from build123d import *

# Parameters (mm, degrees)
SHELL2_T = -1


with BuildPart() as part:
    # Sketch1 → Revolve3 (revolve)
    with BuildSketch(Plane.XY, mode=Mode.PRIVATE) as revolve3_sk:
        with BuildLine():
            Line((0, 0), (70.170274015, 0))
            ThreePointArc((70.170274015, 0), (74.867019818, 0.813696051), (79.016316154, 3.159940352))
            ThreePointArc((79.016316154, 3.159940352), (83.467476244, 7.068955028), (87.638838201, 11.275255219))
            ThreePointArc((87.638838201, 11.275255219), (93.444928024, 16.921383546), (99.811810502, 21.926605983))
            ThreePointArc((99.811810502, 21.926605983), (122.101594507, 34.410654829), (146.474870989, 42.06763466))
            Line((146.474870989, 42.06763466), (146.474870989, 43.043574036))
            Line((146.474870989, 43.043574036), (0, 43.043574036))
            Line((0, 43.043574036), (0, 0))
        make_face()
    revolve(revolve3_sk.sketch.rotate(Axis((0, 43.043574036, 0), (0, -1, 0)), 90), axis=Axis((0, 43.043574036, 0), (0, -1, 0)))

    # Shell2
    shell2_openings = [part.faces().sort_by_distance(p)[0] for p in [
        (0, 43.043574036, 0),
    ]]
    offset(amount=SHELL2_T, openings=shell2_openings, kind=Kind.INTERSECTION)


solid = part.part
Check sheet for the modelled part. Datum: model origin and axes. Units: mm. Give positions to 0.01 mm unless a question says otherwise; leave off trailing zeros. Loops run counter-clockwise (first coordinate to the right, second up) from the corner with the lowest first, then second, coordinate; pieces in that order, holes last. Notation, with made-up numbers: M 60.25,68 L 107.25,68 A30 cw 107.25,105 Z; hole C 38,7 d8. An arc over 180 degrees is marked long. Answer as a JSON object with one key per item and string values. Group by question number.
Q1. Release check for a two-part mould opening along Z. For faces 1 (the flat face through (-1, 0, 1)), 2 (the flat face through (-1, 1, 1)), 3 (the cylindrical face through (-44, 42.56, 139.71)) record: released by +Z, released by -Z, zero draft, split by the parting line, or undercut.
Q2. Cross-section at A-A on y = 32. Record the cut outline in (x, z).
Q3. Material ranges on line 1 along X through (y, z) = (23, 71); line 2 along Y through (x, z) = (27.5, 20.5); line 3 along X through (y, z) = (28, -30.5), recorded low to high. Write a range as [from, to].
Q4. Go/stop test with flat-tipped pins: P1, Ø2, axis at y = 22.5, z = -2, coming from the -X side; P2, Ø12, axis at y = 23.5, z = 0.5, coming from the -X side; P3, Ø3, axis at x = -92.5, z = -92.5, coming from the -Y side. Record where each tip stops, or that it passes through.
Evaluation:
{
 "1": {"face 1": "zero draft", "face 2": "undercut", "face 3": "split by the parting line"},
 "2": {"outline": "C 0,0 d233.71; hole C 0,0 d229.22"},
 "3": {"line 1": "x = [-72.34, -69.85], [69.85, 72.34]", "line 2": "y = [0, 1]", "line 3": "x = [-104.99, -102.92], [102.92, 104.99]"},
 "4": {"P1": "stops at x = -102.08", "P2": "stops at x = -112", "P3": "stops at y = 37.26"}
}
